Solid Edge part; units mm, degrees
sketch "Sketch1" plane through (0, 0, 0) normal (1, 0, 0) x (0, 1, 0)
  line L0 (0, 0) -> (-10, 0)
  line L1 (-10, 0) -> (-10, 6)
  line L2 (-10, 6) -> (-20, 6)
  line L3 (-20, 6) -> (-20, 0)
  line L4 (-20, 0) -> (-23.3082, 0)
  line L5 (-23.3082, -3) -> (-23.3082, 0)
  line L6 (-23.3082, -3) -> (-22, -3)
  line L7 (-22, -3) -> (-22, -5.5)
  line L8 (-22, -5.5) -> (-23.3082, -5.5)
  line L9 (-23.3082, -11.5) -> (-23.3082, -5.5)
  line L10 (-26.6918, -11.5) -> (-23.3082, -11.5)
  line L11 (-26.6918, -5.5) -> (-26.6918, -11.5)
  line L12 (-26.6918, -5.5) -> (-28, -5.5)
  line L13 (-28, -5.5) -> (-28, -3)
  line L14 (-28, -3) -> (-26.6918, -3)
  line L15 (-26.6918, 0) -> (-26.6918, -3)
  line L16 (-26.6918, 0) -> (-30, 0)
  line L17 (-30, 0) -> (-30, 6)
  line L18 (-30, 6) -> (-40, 6)
  line L19 (-40, 6) -> (-40, 0)
  line L20 (-40, 0) -> (-50, 0)
  line L21 (-50, 0) -> (-50, -10)
  line L22 (-10, -54) -> (-50, -10)
  line L23 (0, -54) -> (-10, -54)
  line L24 (0, -43.2) -> (0, -54)
  line L25 (6, -43.2) -> (0, -43.2)
  line L26 (6, -32.4) -> (6, -43.2)
  line L27 (0, -32.4) -> (6, -32.4)
  line L28 (0, -28.6918) -> (0, -32.4)
  line L29 (-3, -28.6918) -> (0, -28.6918)
  line L30 (-3, -28.6918) -> (-3, -30)
  line L31 (-3, -30) -> (-5.5, -30)
  line L32 (-5.5, -30) -> (-5.5, -28.6918)
  line L33 (-11.5, -28.6918) -> (-5.5, -28.6918)
  line L34 (-11.5, -25.3082) -> (-11.5, -28.6918)
  line L35 (-5.5, -25.3082) -> (-11.5, -25.3082)
  line L36 (-5.5, -25.3082) -> (-5.5, -24)
  line L37 (-5.5, -24) -> (-3, -24)
  line L38 (-3, -24) -> (-3, -25.3082)
  line L39 (0, -25.3082) -> (-3, -25.3082)
  line L40 (0, -21.6) -> (0, -25.3082)
  line L41 (6, -21.6) -> (0, -21.6)
  line L42 (6, -10.8) -> (6, -21.6)
  line L43 (0, -10.8) -> (6, -10.8)
  line L44 (0, 0) -> (0, -10.8)
extrude "Protrusion1" add sketch "Sketch1" against normal blind 6
Design review of the part built by this model. Coordinates are the model's own, in mm. A direction names the side the tool comes from. Coordinates: 2 decimals unless noted, no trailing zeros. Write each loop counter-clockwise with the first axis right and the second up, starting at its lowest first coordinate (ties: lowest second). Pieces come first, ordered by that corner, then holes. Notation, with made-up numbers: (-15.75, 69.5) - (-11.75, 69.5) arc R24 cw to (-11.75, 97.5) - close; hole circle Ø1 at (-8.75, 10). An arc over 180 degrees is marked (long way). One line per item, written item: value.
1) Add section B-B (y = -1.5). State the section outline as (x, z) points.
Answer sheet:
outline: (-6, -54) - (0, -54) - (0, -28.69) - (-6, -28.69) - close; (-6, -25.31) - (0, -25.31) - (0, 0) - (-6, 0) - close
2) Add section D-D (z = -46). State the section outline as (x, y) points.
Answer sheet:
outline: (-6, -17.27) - (0, -17.27) - (0, 0) - (-6, 0) - close
3) Add section A-A (z = 2.5). State the section outline as (x, y) points, plus the area to 3 significant figures.
Answer sheet:
outline: (-6, -40) - (0, -40) - (0, -30) - (-6, -30) - close; (-6, -20) - (0, -20) - (0, -10) - (-6, -10) - close
area: 120 mm2
4) Insertion check: pin 1 (1 mm diameter, centred on x = -2.5, z = -27.5, fed in from +Y); pin 2 (6 mm diameter, centred on y = -18, z = -8, fed in from +X); pin 3 (0.7 mm diameter, centred on x = -2.5, z = -25, fed in from -Y); pin 4 (1.8 mm diameter, centred on x = -1.5, z = 2.5, fed in from -Y). Each pin has a flat end and moves straight along its axis. Give the tip position at first contact, or say it passes through.
Answer sheet:
pin 1: stops at y = -11.5
pin 2: stops at x = 0
pin 3: stops at y = -36.68
pin 4: stops at y = -40
5) Mouldability with a two-part tool opening along Z and no side actions: class faces 1 (the face through (-3, -28, -4)), 2 (the face through (-3, -22, 0)), 3 (the face through (-3, -23.308, -9)) as +Z half, -Z half, draft (parallel to the pull), parting line (faces both ways), or undercut.
Answer sheet:
face 1: undercut
face 2: +Z half
face 3: draft
6) For faces 4 (the face through (-3, -4, -30)), 5 (the face through (-3, -2, -28.692)), 6 (the face through (-3, -5, 0)), list the 3-axis set-ups (+Z, -Z, +X, -X, +Y, -Y) from which the entire face can be reached by the end or side of a thin tool; tool diameter is ignored.
Answer sheet:
face 4: +X, -X
face 5: +X, -X, +Y
face 6: +Z, +X, -X, +Y
7) To check wall thickness, follow probe 1 along Y at (x, z) = (-1.5, -4); probe 2 along Z at (x, y) = (-1.85, -0.5); probe 3 along Y at (x, z) = (-1.8, -8). State the ranges of each line that lie inside material, in increasing order.
Answer sheet:
probe 1: y = -50 to -28, -22 to 0
probe 2: z = -54 to -28.69, -25.31 to 0
probe 3: y = -50 to -26.69, -23.31 to 0
8) Add section C-C (y = -41.5). State the section outline as (x, z) points, plus the area to 3 significant figures.
Answer sheet:
outline: (-6, -19.35) - (0, -19.35) - (0, 0) - (-6, 0) - close
area: 116 mm2
